For this review, take the finished solid that the model builds, in its own axes (mm). Face numbers are marked on the shaded views. Coordinates: 2 decimals unless noted, no trailing zeros. Loops run counter-clockwise (first coordinate to the right, second up) from the corner with the lowest first, then second, coordinate; pieces in that order, holes last. Notation, with made-up numbers: M 38.25,-5 L 48.25,-5 A30 cw 48.25,24 Z; hole C 32,7 d3. An arc over 180 degrees is marked long. Write item = value, one per line.
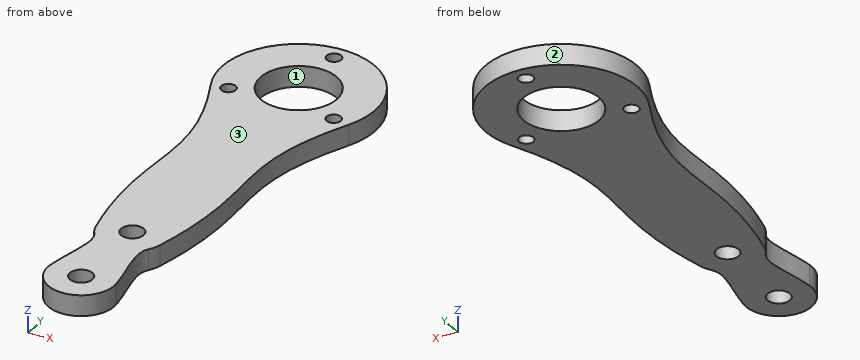
from build123d import *

# Parameters (mm, degrees)
SKETCH1_R           = 2.1
SKETCH1_R_2         = 11
SKETCH1_R_3         = 3.2639
BOSS_EXTRUDE1_DEPTH = 6


with BuildPart() as part:
    # Sketch1 → Boss-Extrude1 (new body)
    with BuildSketch(Plane.XY):
        with BuildLine():
            ThreePointArc((19.889218642, 15.996863194), (0, 47.4), (-19.889218642, 15.996863194))
            add(Edge.make_bspline(
                [(-19.889218642, 15.996863194), (-3.976229329, -17.66179032), (-18.147711497, -22.281552166), (-9.262906138, -59.369052697)],
                knots=[0, 0, 0, 0, 1, 1, 1, 1], degree=3))
            ThreePointArc((-9.262906138, -59.369052697), (-8.692742138, -61.0438232), (-7.822687238, -62.584260701))
            add(Edge.make_bspline(
                [(-9.462887275, -81.464003027), (-8.561282023, -73.607821952), (-5.270691934, -66.257890325), (-7.822687238, -62.584260701)],
                knots=[0, 0, 0, 0, 1, 1, 1, 1], degree=3))
            ThreePointArc((-9.462887275, -81.464003027), (0, -92.075), (9.462887275, -81.464003027))
            add(Edge.make_bspline(
                [(9.462887275, -81.464003027), (8.561282023, -73.607821952), (5.270691934, -66.257890325), (7.822687238, -62.584260701)],
                knots=[0, 0, 0, 0, 1, 1, 1, 1], degree=3))
            ThreePointArc((7.822687238, -62.584260701), (8.692742138, -61.0438232), (9.262906138, -59.369052697))
            add(Edge.make_bspline(
                [(19.889218642, 15.996863194), (3.976229329, -17.66179032), (18.147711497, -22.281552166), (9.262906138, -59.369052697)],
                knots=[0, 0, 0, 0, 1, 1, 1, 1], degree=3))
        make_face()
        with Locations((-15.155444566, 16.65)):
            Circle(SKETCH1_R, mode=Mode.SUBTRACT)
        with Locations((0, 42.9)):
            Circle(SKETCH1_R, mode=Mode.SUBTRACT)
        with Locations((0, 25.4)):
            Circle(SKETCH1_R_2, mode=Mode.SUBTRACT)
        with Locations((15.155444566, 16.65)):
            Circle(SKETCH1_R, mode=Mode.SUBTRACT)
        with Locations((0, -57.15)):
            Circle(SKETCH1_R_3, mode=Mode.SUBTRACT)
        with Locations((0, -82.55)):
            Circle(SKETCH1_R_3, mode=Mode.SUBTRACT)
    extrude(amount=BOSS_EXTRUDE1_DEPTH)


solid = part.part
Q1. For pin 1 Ø1.5 at (y, z) = (30, 4.5) entering from +X; pin 2 Ø1.5 at (x, z) = (-7.5, 2) entering from -Y; pin 3 Ø1 at (x, z) = (8.5, 3) entering from +Y, all flat-tipped, find the tip position at first contact; note any pin that passes through.
Solved:
pin_1 = 21.66
pin_2 = -89.27
pin_3 = 45.89
Q2. For line 1 along Y through (x, z) = (0, 1.9) (3 decimals); line 2 along X through (y, z) = (30.5, 1); line 3 along Y through (x, z) = (3.5, 3), list the stretches that pass through material, from the lowest coordinate up.
Solved:
line_1 = -92.075 to -85.814, -79.286 to -60.414, -53.886 to 14.4, 36.4 to 40.8, 45 to 47.4
line_2 = -21.4 to -9.75, 9.75 to 21.4
line_3 = -91.41 to 14.97, 35.83 to 47.12
Q3. Draft analysis for pull direction Y (two halves, no side actions). For the marked faces 1, 2 and 3, state which applies: +Y half, -Y half, draft (parallel to the pull), parting line (faces both ways), or undercut.
Solved:
face_1 = undercut
face_2 = parting line
face_3 = draft
Q4. Add section C-C (y = 42.9). Write out the cut boundary in (x, z).
Solved:
outline = M -13.33,0 L -2.1,0 L -2.1,6 L -13.33,6 Z; M 2.1,0 L 13.33,0 L 13.33,6 L 2.1,6 Z
Q5. Add section A-A (y = 25.4). Write out the cut boundary in (x, z), and give its area (3 significant figures).
Solved:
outline = M -22,0 L -11,0 L -11,6 L -22,6 Z; M 11,0 L 22,0 L 22,6 L 11,6 Z
area = 132 mm²
Q6. Add section B-B (z = 4). State how many separate pieces and enclosed holes the cut face has, and give its area (3 significant figures).
Solved:
separate_pieces = 1
enclosed_holes = 6
area = 3,130 mm²
